Here's how the part is built. I have some questions about the finished solid (model axes, mm). Round coordinates to 2 decimals unless told otherwise and drop trailing zeros. Loops run counter-clockwise (first coordinate to the right, second up) from the corner with the lowest first, then second, coordinate; pieces in that order, holes last. Notation, with made-up numbers: M 26,21 L 57,21 A36 cw 57,55 Z; hole C 3,48 d8. An arc over 180 degrees is marked long. Answer as a JSON object with one key per item and string values.
from build123d import *

# Parameters (mm, degrees)
SKETCH_1_W          = 10
SKETCH_1_H          = 30
SKETCH_1_W_2        = 8
SKETCH_1_H_2        = 28
EXTRUDE_1_DEPTH     = 700
SKETCH_2_R          = 1.6
CUT_EXTRUDE_1_DEPTH = 701.660402763
SKETCH_3_R          = 10
CUT_EXTRUDE_2_DEPTH = 701.232104377


with BuildPart() as part:
    # ｽｹｯﾁ1 → 押し出し-薄板1 (new body)
    with BuildSketch(Plane.XY):
        Rectangle(SKETCH_1_W, SKETCH_1_H)
        Rectangle(SKETCH_1_W_2, SKETCH_1_H_2, mode=Mode.SUBTRACT)
    extrude(amount=EXTRUDE_1_DEPTH)

    # ｽｹｯﾁ2 → ｶｯﾄ - 押し出し1 (cut, through all)
    with BuildSketch(Plane(origin=(0, 15, 0), x_dir=(1, 0, 0), z_dir=(0, 1, 0))):
        with Locations(Location((0, -5, 0), (0, 0, 270))):
            Circle(SKETCH_2_R)
        with Locations(Location((0, -110, 0), (0, 0, 270))):
            Circle(SKETCH_2_R)
        with Locations(Location((0, -695, 0), (0, 0, 90))):
            Circle(SKETCH_2_R)
        with Locations(Location((0, -590, 0), (0, 0, 90))):
            Circle(SKETCH_2_R)
    extrude(amount=-CUT_EXTRUDE_1_DEPTH, mode=Mode.SUBTRACT)

    # ｽｹｯﾁ3 → ｶｯﾄ - 押し出し2 (cut, through all)
    with BuildSketch(Plane(origin=(5, 0, 0), x_dir=(0, 0, -1), z_dir=(1, 0, 0))):
        with Locations((-677.5, 0)):
            Circle(SKETCH_3_R)
        with Locations((-652.5, 0)):
            Circle(SKETCH_3_R)
        with Locations((-627.5, 0)):
            Circle(SKETCH_3_R)
        with Locations((-602.5, 0)):
            Circle(SKETCH_3_R)
        with Locations((-577.5, 0)):
            Circle(SKETCH_3_R)
        with Locations((-552.5, 0)):
            Circle(SKETCH_3_R)
        with Locations((-527.5, 0)):
            Circle(SKETCH_3_R)
        with Locations((-502.5, 0)):
            Circle(SKETCH_3_R)
        with Locations((-477.5, 0)):
            Circle(SKETCH_3_R)
        with Locations((-452.5, 0)):
            Circle(SKETCH_3_R)
    extrude(amount=-CUT_EXTRUDE_2_DEPTH, mode=Mode.SUBTRACT)


solid = part.part
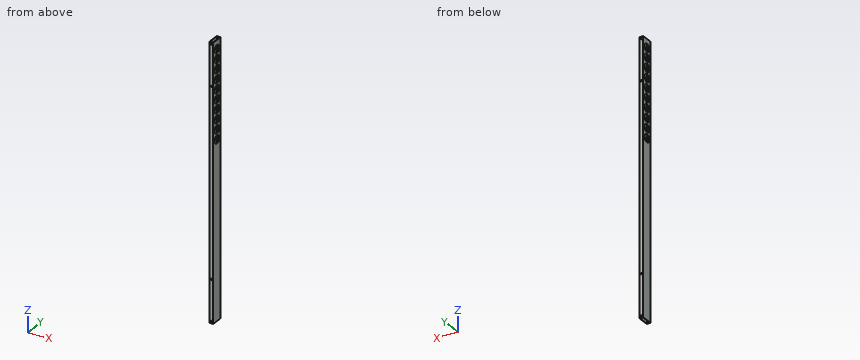
Item 1: Please list where these lines run through material, in increasing order: probe 1 along Y at (x, z) = (-4.25, 502.5); probe 2 along X at (y, z) = (-2.5, 71.5); probe 3 along Y at (x, z) = (0, 661.5). Write a range as from..to.
Resolved:
{"probe 1": "-15..-10, 10..15", "probe 2": "-5..-4, 4..5", "probe 3": "-15..-14, 14..15"}
Item 2: I want a section at A-A, the plane z = 577.5. Please give me the cut outline in (x, y).
Resolved:
{"outline": "M -5,-15 L 5,-15 L 5,-10 L 4,-10 L 4,-14 L -4,-14 L -4,-10 L -5,-10 Z; M -5,10 L -4,10 L -4,14 L 4,14 L 4,10 L 5,10 L 5,15 L -5,15 Z"}
Item 3: I want a section at C-C, the plane x = 0. State how many separate pieces and enclosed holes the cut face has, then the cut area to 3 significant figures.
Resolved:
{"separate pieces": "10", "enclosed holes": "0", "area": "1,370 mm²"}
Item 4: I want a section at D-D, the plane z = 450. Please give me the cut outline in (x, y), then the cut area to 3 significant figures.
Resolved:
{"outline": "M -5,-15 L 5,-15 L 5,-9.68 L 4,-9.68 L 4,-14 L -4,-14 L -4,-9.68 L -5,-9.68 Z; M -5,9.68 L -4,9.68 L -4,14 L 4,14 L 4,9.68 L 5,9.68 L 5,15 L -5,15 Z", "area": "37.3 mm²"}
Item 5: I want a section at B-B, the plane z = 211.5. Please give me the cut outline in (x, y).
Resolved:
{"outline": "M -5,-15 L 5,-15 L 5,15 L -5,15 Z; hole M -4,-14 L 4,-14 L 4,14 L -4,14 Z"}
Item 6: I'm going to push flat-ended pins straight in: pin 1 Ø12 at (y, z) = (0, 477.5) entering from -X; pin 2 Ø5 at (x, z) = (0, 5) entering from +Y. Where does each tip first touch, or does it pass through?
Resolved:
{"pin 1": "through", "pin 2": "y = 15"}
